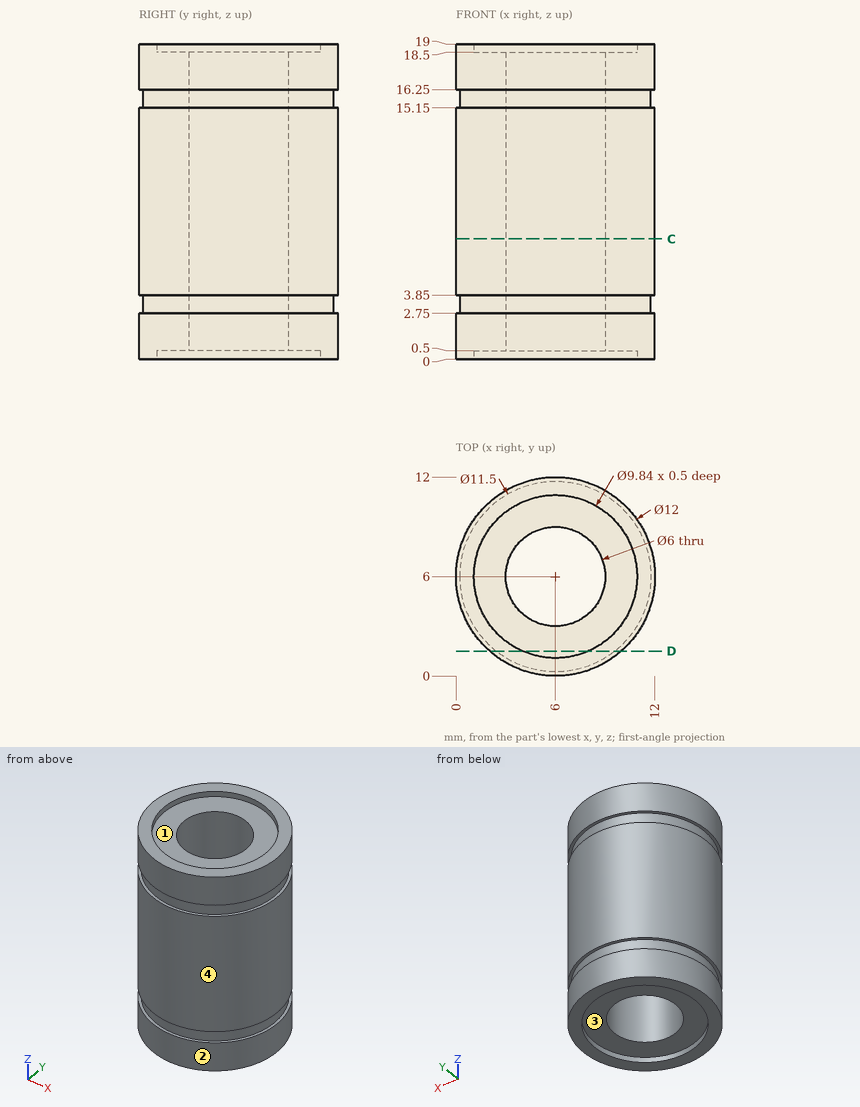
Input: dimensioned drawing with shaded views. Units: mm. Origin: part minimum x, y, z. A direction names the side the tool comes from. Round coordinates to 2 decimals unless told otherwise and drop trailing zeros. Order: outer loops, then holes, each group sorted by start corner. A loop starts at its lowest first (then second) coordinate and runs counter-clockwise, first axis right, second up. Notation, with made-up numbers: (49.25, 79.5) - (75.25, 79.5) arc R9 cw to (75.25, 91.5) - close; hole circle Ø7 at (42.5, 66). An arc over 180 degrees is marked (long way). Answer as a JSON object with one key per item and string values. Group by question number.
(1) Pin query (flat end, axial travel): P1, Ø4, axis at x = 10.5, z = 7, coming from the +Y side; P2, Ø6, axis at y = 10, z = 10, coming from the -X side; P3, Ø6, axis at x = 6.5, y = 7.5, coming from the -Z side; P4, Ø3, axis at x = 5, y = 5, coming from the +Z side. Return the tip coordinate at first contact, or that it passes through.
(2) Cut plane C-C (z = 7.25). Return loops of the section in (x, y).
(3) Draft query along Y for the marked faces 3 and 4. Return one class per face: released by +Y, released by -Y, zero draft, split by the parting line, or undercut.
(4) Reachability of the marked faces 1 and 2 from +Z, -Z, +X, -X, +Y, -Y: full face, straight path, thin tool, end or side. Return the list, or none.
(5) Cut plane D-D (y = 1.5). Return loops of the section in (x, z), then the cut area to 3 significant figures.
(6) Material intervals for probe 1 along Y at (x, z) = (6, 18.75); probe 2 along Y at (x, z) = (6, 14); probe 3 along Z at (x, y) = (10, 4.75), sorted ascending. Write a range as from..to.
Here are the results:
{
 "1": {"P1": "stops at y = 11.45", "P2": "stops at x = 0.08", "P3": "stops at z = 0.5", "P4": "passes through"},
 "2": {"outline": "circle Ø12 at (6, 6); hole circle Ø6 at (6, 6)"},
 "3": {"face 3": "undercut", "face 4": "split by the parting line"},
 "4": {"face 1": "+Z", "face 2": "+Z, -Z"},
 "5": {"outline": "(2.03, 0) - (4.01, 0) - (4.01, 0.5) - (7.99, 0.5) - (7.99, 0) - (9.97, 0) - (9.97, 2.75) - (9.58, 2.75) - (9.58, 3.85) - (9.97, 3.85) - (9.97, 15.15) - (9.58, 15.15) - (9.58, 16.25) - (9.97, 16.25) - (9.97, 19) - (7.99, 19) - (7.99, 18.5) - (4.01, 18.5) - (4.01, 19) - (2.03, 19) - (2.03, 16.25) - (2.42, 16.25) - (2.42, 15.15) - (2.03, 15.15) - (2.03, 3.85) - (2.42, 3.85) - (2.42, 2.75) - (2.03, 2.75) - close", "area": "145 mm^2"},
 "6": {"probe 1": "y = 0..1.08, 10.92..12", "probe 2": "y = 0..3, 9..12", "probe 3": "z = 0.5..18.5"}
}
